Job drawing, mm, ordinate dimensions from the low corner. One solid piece. A direction names the side the tool comes from. Give positions to 0.01 mm unless a question says otherwise; leave off trailing zeros. Order: outer loops, then holes, each group sorted by start corner. A loop starts at its lowest first (then second) coordinate and runs counter-clockwise, first axis right, second up. Notation, with made-up numbers: (15, -39.75) -> (68, -39.75) arc R5 ccw to (68, -33.75) -> close; hole circle Ø8 at (-27, 9). An arc over 180 degrees is marked (long way). Write item = value, one per line. Start each with the question number.
(1) Two-plate mould, pull along Z, no slides. Class the marked faces 1, 2 and 3: pulls with the +Z half, pulls with the -Z half, needs draft (parallel to the pull), parting line crosses it, or undercut.
(2) Saw through at A-A, the plane z = 12.25. List the corners of the cut face in (x, y).
(3) Which spindle directions (+Z, -Z, +X, -X, +Y, -Y) get a long thin tool onto all of the face, cutting with end or side? Do the marked faces 4 and 5. Say none if no direction does.
(4) Saw through at B-B, the plane x = 8.25. List the corners of the cut face in (y, z), then the cut area to 3 significant figures.
(5) Saw through at D-D, the plane y = 2.8. List the corners of the cut face in (x, z).
(6) Flat gauge pins, fed straight in: pin 1 (4 mm diameter, centred on x = 8.5, z = 2.5, fed in from +Y); pin 2 (1 mm diameter, centred on y = 1, z = 5.5, fed in from -X). Where does each tip first touch, or does it go through?
(7) Probe line 1 along X through (y, z) = (3.25, 8); line 2 along Y through (x, z) = (1, 5.5); line 3 along X through (y, z) = (1.4, 6.25). List the from-to ranges inside material, lowest first. Write a range as from..to.
(8) Saw through at C-C, the plane z = 8.25. List the corners of the cut face in (x, y), then the cut area to 3 significant figures.
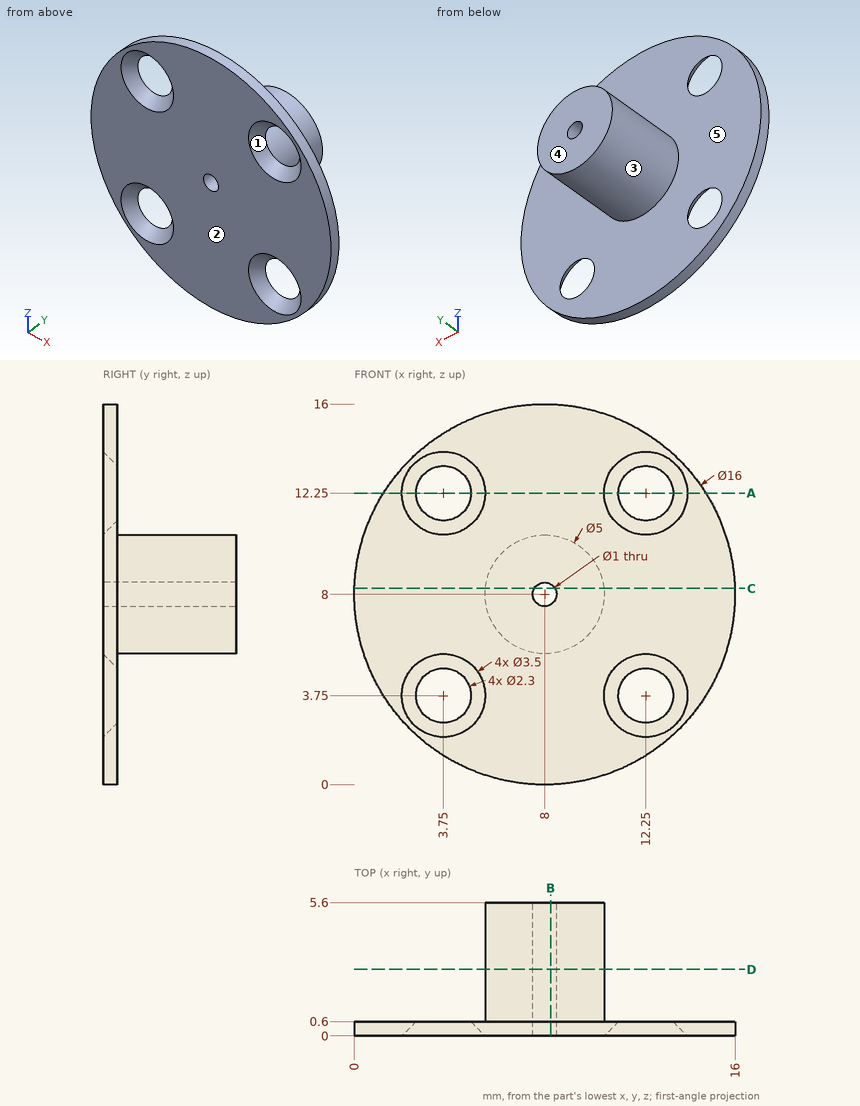
Results list:
q1.face_1 = undercut
q1.face_2 = needs draft
q1.face_3 = parting line crosses it
q2.outline = (1.22, 0) -> (2, 0) -> (2.6, 0.6) -> (1.22, 0.6) -> close; (4.9, 0.6) -> (5.5, 0) -> (10.5, 0) -> (11.1, 0.6) -> close; (13.4, 0.6) -> (14, 0) -> (14.78, 0) -> (14.78, 0.6) -> close
q3.face_4 = +Z, -Z, +X, -X, +Y
q3.face_5 = +Y
q4.outline = (0, 0) -> (0.6, 0) -> (0.6, 5.51) -> (5.6, 5.51) -> (5.6, 7.57) -> (0, 7.57) -> close; (0, 8.43) -> (5.6, 8.43) -> (5.6, 10.49) -> (0.6, 10.49) -> (0.6, 16) -> (0, 16) -> close
q4.area = 29.6 mm^2
q5.outline = circle Ø5 at (8, 8); hole circle Ø1 at (8, 8)
q6.pin_1 = 0.6
q6.pin_2 = 0.31
q7.line_1 = 5.5..7.5, 8.5..10.5
q7.line_2 = 0..0.6
q7.line_3 = 6.21..9.79
q8.outline = (0, 0) -> (7.57, 0) -> (7.57, 5.6) -> (5.51, 5.6) -> (5.51, 0.6) -> (0, 0.6) -> close; (8.43, 0) -> (16, 0) -> (16, 0.6) -> (10.49, 0.6) -> (10.49, 5.6) -> (8.43, 5.6) -> close
q8.area = 29.6 mm^2
